Check sheet for the drawn part. Datum: minimum x, y, z corner. Units: mm. Give positions to 0.01 mm unless a question says otherwise; leave off trailing zeros. Write each loop counter-clockwise with the first axis right and the second up, starting at its lowest first coordinate (ties: lowest second). Pieces come first, ordered by that corner, then holes. Notation, with made-up numbers: (-9.75, 80) - (2.25, 80) arc R21 ccw to (2.25, 92) - close; hole circle Ø7 at (40.25, 85.5). An arc over 180 degrees is marked (long way). Use a Markdown table: item, result.
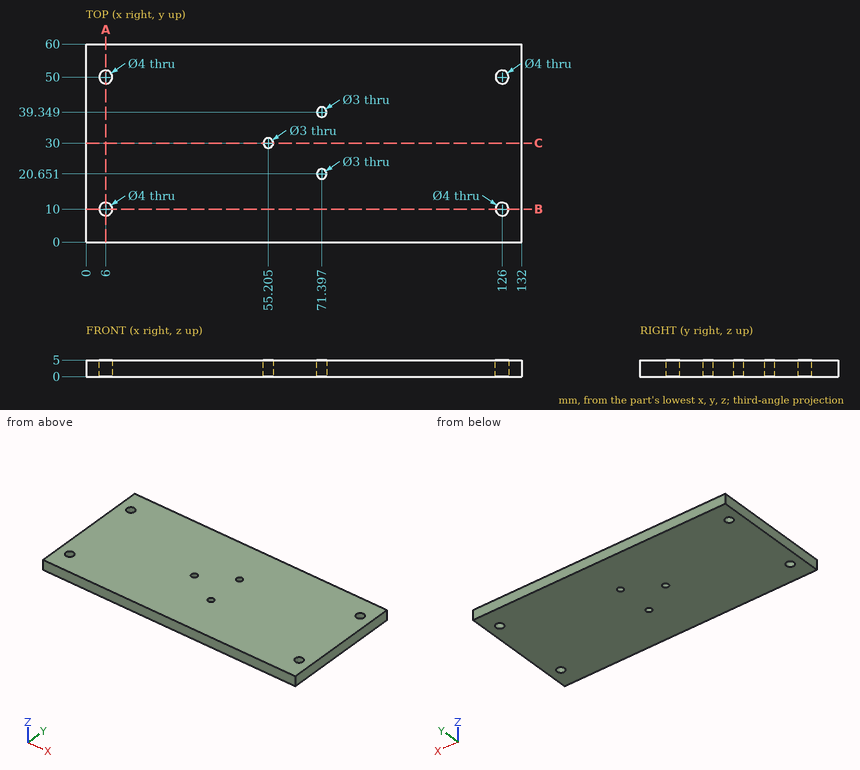
1) Depth check by flat-ended pin: P1, Ø1.8, axis at x = 71.4, y = 20.65, coming from the -Z side (3 decimals). Enter the tip coordinate at first touch or a pass-through.
Working result:
| item | result |
|---|---|
| P1 | passes through |
2) Section check A-A on x = 6. Record the boundary of the cut face in (y, z).
Working result:
| item | result |
|---|---|
| outline | (0, 0) - (8, 0) - (8, 5) - (0, 5) - close; (12, 0) - (48, 0) - (48, 5) - (12, 5) - close; (52, 0) - (60, 0) - (60, 5) - (52, 5) - close |
3) Section check C-C on y = 30. Record the boundary of the cut face in (x, z) (1 decimal).
Working result:
| item | result |
|---|---|
| outline | (0, 0) - (53.7, 0) - (53.7, 5) - (0, 5) - close; (56.7, 0) - (132, 0) - (132, 5) - (56.7, 5) - close |
4) Material ranges on L1, parallel to Y at x = 126, z = 4.05; L2, parallel to X at y = 20.5, z = 1 (1 decimal); L3, parallel to X at y = 29, z = 2.7 (1 decimal), recorded low to high. Write a range as from..to.
Working result:
| item | result |
|---|---|
| L1 | y = 0..8, 12..48, 52..60 |
| L2 | x = 0..69.9, 72.9..132 |
| L3 | x = 0..54.1, 56.3..132 |
5) Section check B-B on y = 10. Record the boundary of the cut face in (x, z), then the cut area to 3 significant figures.
Working result:
| item | result |
|---|---|
| outline | (0, 0) - (4, 0) - (4, 5) - (0, 5) - close; (8, 0) - (124, 0) - (124, 5) - (8, 5) - close; (128, 0) - (132, 0) - (132, 5) - (128, 5) - close |
| area | 620 mm² |
